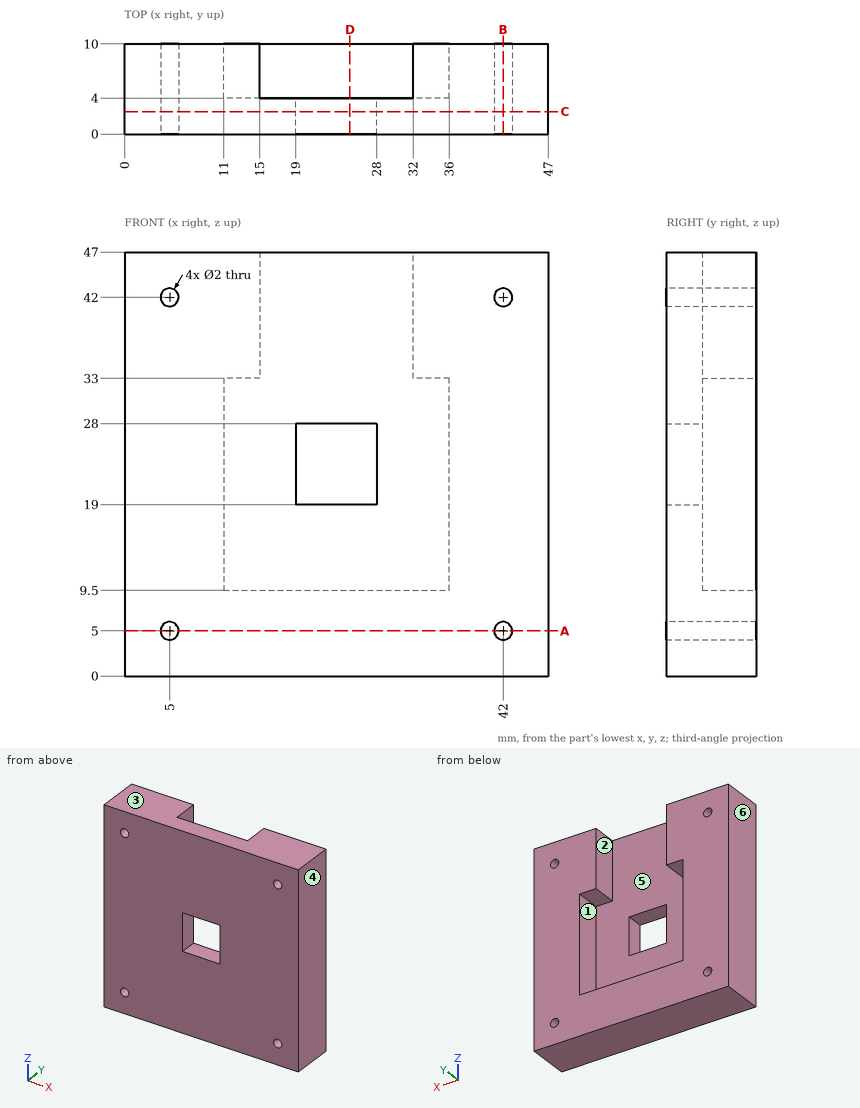
Design review of the part shown in the three views and the two pictorial views. Dimensions are in mm from the part's minimum x, y and z. A direction names the side the tool comes from. Round coordinates to 2 decimals unless told otherwise and drop trailing zeros. Write each loop counter-clockwise with the first axis right and the second up, starting at its lowest first coordinate (ties: lowest second). Pieces come first, ordered by that corner, then holes. Notation, with made-up numbers: (-36, 27.5) -> (-8, 27.5) arc R17 ccw to (-8, 46.5) -> close; hole circle Ø7 at (32.5, 2). An arc over 180 degrees is marked (long way). Write item = value, one per line. Start each with the question number.
1) Mouldability with a two-part tool opening along X and no side actions: class the marked faces 4, 5 and 6 as +X half, -X half, draft (parallel to the pull), parting line (faces both ways), or undercut.
2) Take a section at C-C, the plane y = 2.5. State the section outline as (x, z) points, plus the area to 3 significant figures.
3) Tool access review of the marked faces 1, 2 and 3: name each direction out of +Z, -Z, +X, -X, +Y, -Y from which nothing blocks a thin tool from reaching the whole face with its end or side.
4) Take a section at B-B, the plane x = 42. State the section outline as (y, z) points, plus the area to 3 significant figures.
5) Wall thickness on probe 1 along X at (y, z) = (2, 42); probe 2 along X at (y, z) = (5, 42); probe 3 along X at (y, z) = (6, 38): over which ranges is each line inside the solid? List them lowest first. Write a range as from..to.
6) Clearance check with flat-ended pins moving along their axes: pin 1 (1.8 mm diameter, centred on x = 23, y = 8, fed in from +Z); pin 2 (8 mm diameter, centred on x = 19.5, z = 18.5, fed in from +Y). State where each tip first meets the part, or that it passes through.
7) Take a section at A-A, the plane z = 5. State the section outline as (x, y) points.
8) Take a section at D-D, the plane x = 25. State the section outline as (y, z) points.
Results list:
q1.face_4 = +X half
q1.face_5 = undercut
q1.face_6 = -X half
q2.outline = (0, 0) -> (47, 0) -> (47, 47) -> (0, 47) -> close; hole circle Ø2 at (5, 5); hole circle Ø2 at (5, 42); hole (19, 19) -> (28, 19) -> (28, 28) -> (19, 28) -> close; hole circle Ø2 at (42, 5); hole circle Ø2 at (42, 42)
q2.area = 2,120 mm²
q3.face_1 = +Y
q3.face_2 = +Z, +Y
q3.face_3 = +Z, +X, -X, +Y, -Y
q4.outline = (0, 0) -> (10, 0) -> (10, 4) -> (0, 4) -> close; (0, 6) -> (10, 6) -> (10, 41) -> (0, 41) -> close; (0, 43) -> (10, 43) -> (10, 47) -> (0, 47) -> close
q4.area = 430 mm²
q5.probe_1 = 0..4, 6..41, 43..47
q5.probe_2 = 0..4, 6..15, 32..41, 43..47
q5.probe_3 = 0..15, 32..47
q6.pin_1 = 9.5
q6.pin_2 = 4
q7.outline = (0, 0) -> (4, 0) -> (4, 10) -> (0, 10) -> close; (6, 0) -> (41, 0) -> (41, 10) -> (6, 10) -> close; (43, 0) -> (47, 0) -> (47, 10) -> (43, 10) -> close
q8.outline = (0, 0) -> (10, 0) -> (10, 9.5) -> (4, 9.5) -> (4, 19) -> (0, 19) -> close; (0, 28) -> (4, 28) -> (4, 47) -> (0, 47) -> close
